```python
from build123d import *

# Parameters (mm, degrees)
SKETCH2_W                    = 44
SKETCH2_H                    = 12
SKETCH2_R                    = 2.7
BASE_FLANGE1_DEPTH           = 3
EDGE_FLANGE1_STRIP_W         = 13.4732
EDGE_FLANGE1_STRIP_H         = 3
EDGE_FLANGE1_STRIP_CUT_DEPTH = 44
EDGE_FLANGE1_DEPTH           = 44
CUT_EXTRUDE1_DEPTH           = 10
SKETCH11_R                   = 8.1
CUT_EXTRUDE2_DEPTH           = 10


# Sheet-metal steps are written as plain solids
with BuildPart() as part:
    # Sketch2 → Base-Flange1 (new body)
    with BuildSketch(Plane.XY):
        with Locations((22, -6)):
            Rectangle(SKETCH2_W, SKETCH2_H)
        with Locations((5.5, -6)):
            Circle(SKETCH2_R, mode=Mode.SUBTRACT)
        with Locations((38.5, -6)):
            Circle(SKETCH2_R, mode=Mode.SUBTRACT)
    extrude(amount=-BASE_FLANGE1_DEPTH)

    # Edge-Flange1 strip (across the edge) → Edge-Flange1 strip cut (cut)
    with BuildSketch(Plane(origin=(44, 0, 0), x_dir=(0, -1, 0), z_dir=(-1, 0, 0))):
        with Locations((-6, -1.5)):
            Rectangle(EDGE_FLANGE1_STRIP_W, EDGE_FLANGE1_STRIP_H)
    extrude(amount=EDGE_FLANGE1_STRIP_CUT_DEPTH, mode=Mode.SUBTRACT)

    # Edge-Flange1 section (across the edge) → Edge-Flange1 (add)
    with BuildSketch(Plane(origin=(44, 0, 0), x_dir=(0, -1, 0), z_dir=(-1, 0, 0))):
        with BuildLine():
            Line((-3, 0.7366), (-3, 29.1))
            Line((-3, 29.1), (0, 29.1))
            Line((0, 29.1), (0, 0.7366))
            ThreePointArc((0, 0.7366), (0.215745145, 0.215745145), (0.7366, 0))
            Line((0.7366, 0), (0.7366, -3))
            ThreePointArc((0.7366, -3), (-1.905575199, -1.905575199), (-3, 0.7366))
        make_face()
    extrude(amount=EDGE_FLANGE1_DEPTH)

    # Sketch10 → Cut-Extrude1 (cut)
    with BuildSketch(Plane.XZ):
        with BuildLine():
            Line((0, 0.7366), (13.527598835, 22.312101137))
            ThreePointArc((13.527598835, 22.312101137), (22, 27), (30.472401165, 22.312101137))
            Line((30.472401165, 22.312101137), (44, 0.7366))
            Line((44, 0.7366), (48.421398218, 0.7366))
            Line((48.421398218, 0.7366), (48.421398218, 35.108579441))
            Line((48.421398218, 35.108579441), (-4.285342107, 35.108579441))
            Line((-4.285342107, 35.108579441), (-4.285342107, 0.7366))
            Line((-4.285342107, 0.7366), (0, 0.7366))
        make_face()
    extrude(amount=-CUT_EXTRUDE1_DEPTH, mode=Mode.SUBTRACT)

    # Sketch11 → Cut-Extrude2 (cut)
    with BuildSketch(Plane.XZ):
        with Locations(Location((22, 17, 0), (0, 0, 270))):
            Circle(SKETCH11_R)
    extrude(amount=-CUT_EXTRUDE2_DEPTH, mode=Mode.SUBTRACT)


solid = part.part
```
Verification items for the finished model (mm, model axes). A direction names the side the tool comes from. Coordinates: 2 decimals unless noted, no trailing zeros. Write each loop counter-clockwise with the first axis right and the second up, starting at its lowest first coordinate (ties: lowest second). Pieces come first, ordered by that corner, then holes. Notation, with made-up numbers: M 3.5,79.25 L 19.5,79.25 A20 cw 19.5,102.25 Z; hole C 25.5,-21 d5. An arc over 180 degrees is marked long. Answer as a JSON object with one key per item and string values. Group by question number.
(1) Cross-section at A-A, the plane y = -6. Record the cut outline in (x, z).
(2) Gauge pin test, flat ends, axial feed: pin 1 (1 mm diameter, centred on x = 16.5, z = 7, fed in from -Y); pin 2 (6 mm diameter, centred on x = 5.5, y = -6, fed in from -Z); pin 3 (4 mm diameter, centred on x = 37, y = -1, fed in from +Z); pin 4 (1 mm diameter, centred on y = 1, z = 19, fed in from -X). Record the tip position at first contact, or that the pin passes through.
(3) Release check for a two-part mould opening along X. For faces 3 (the face through (41.075, -5.189, -1.479)), 4 (the face through (17.071, 1.479, 23.428)), 5 (the face through (6.669, 1.479, 11.373)), 6 (the face through (22, 0, 8)) record: +X half, -X half, draft (parallel to the pull), parting line (faces both ways), or undercut.
(4) Cross-section at D-D, the plane y = -4. Record the cut outline in (x, z).
(5) Tool access check on faces 1 (the face through (44, -5, -2)), 2 (the face through (22, -6, 0)). Record the directions out of +Z, -Z, +X, -X, +Y, -Y that give a thin tool (end or side, any length) a straight path to the whole face; none if there is none.
(6) Cross-section at C-C, the plane z = 11.5. Record the cut outline in (x, y), and give its area (3 significant figures).
(7) Cross-section at B-B, the plane x = 22. Record the cut outline in (y, z).
(8) Material ranges on line 1 (Y direction, x = 7, z = 3); line 2 (Z direction, x = 26, y = -3.75); line 3 (Y direction, x = 5.5, z = -2.05), recorded low to high.
Reply:
{
 "1": {"outline": "M 0,-3 L 2.8,-3 L 2.8,0 L 0,0 Z; M 8.2,-3 L 35.8,-3 L 35.8,0 L 8.2,0 Z; M 41.2,-3 L 44,-3 L 44,0 L 41.2,0 Z"},
 "2": {"pin 1": "y = 0", "pin 2": "z = -3", "pin 3": "z = 14.66", "pin 4": "x = 11.14"},
 "3": {"face 3": "undercut", "face 4": "undercut", "face 5": "-X half", "face 6": "draft"},
 "4": {"outline": "M 0,-3 L 3.69,-3 L 3.69,0 L 0,0 Z; M 7.31,-3 L 36.69,-3 L 36.69,0 L 7.31,0 Z; M 40.31,-3 L 44,-3 L 44,0 L 40.31,0 Z"},
 "5": {"face 1": "+Z, -Z, +X, +Y, -Y", "face 2": "+Z, +X, -X, -Y"},
 "6": {"outline": "M 6.75,0 L 16.05,0 L 16.05,3 L 6.75,3 Z; M 27.95,0 L 37.25,0 L 37.25,3 L 27.95,3 Z", "area": "55.8 mm²"},
 "7": {"outline": "M -12,-3 L -0.74,-3 A3.74 ccw 3,0.74 L 3,8.9 L 0,8.9 L 0,0.74 A0.74 cw -0.74,0 L -12,0 Z; M 0,25.1 L 3,25.1 L 3,27 L 0,27 Z"},
 "8": {"line 1": "0 to 3", "line 2": "-3 to 0", "line 3": "-12 to -8.7, -3.3 to 1.75"}
}
